Can you work these out from the drawing? Everything is in mm from the part's minimum corner. A direction names the side the tool comes from. Give positions to 0.01 mm unless a question says otherwise; leave off trailing zeros. Write each loop counter-clockwise with the first axis right and the second up, starting at its lowest first coordinate (ties: lowest second). Pieces come first, ordered by that corner, then holes. Notation, with made-up numbers: (71.5, -10) -> (99.5, -10) arc R26 ccw to (99.5, 21) -> close; hole circle Ø2 at (-14, 19.5). An arc over 180 degrees is marked (long way). Return JSON: item names as keys, results as strings.
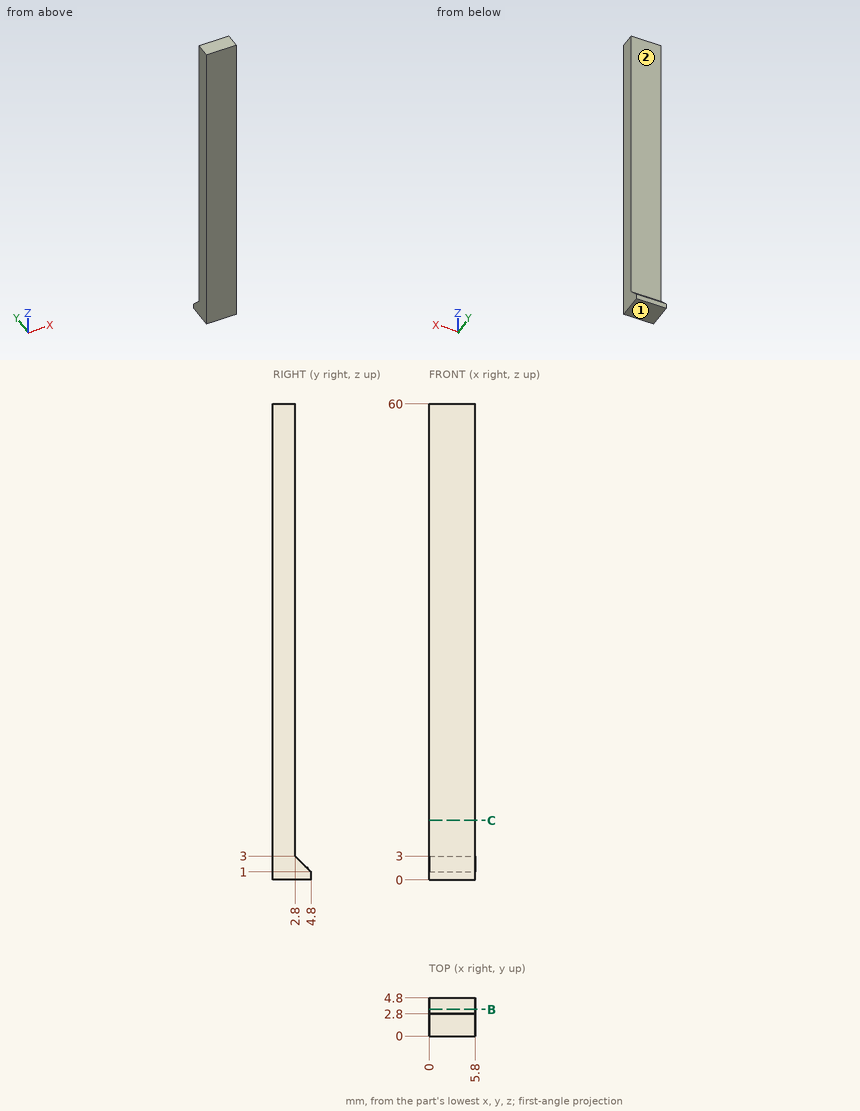
1. Suppose I cut it at B-B, the plane y = 3.35. List the corners of the cut face in (x, z) for me, and give its area (3 significant figures).
Taken from the geometry:
{"outline": "(0, 0) -> (5.8, 0) -> (5.8, 2.45) -> (0, 2.45) -> close", "area": "14.2 mm²"}
2. If I drill on line 1 (Y direction, x = 5.25, z = 41); line 2 (Z direction, x = 3.8, y = 4.65), over which ranges is the centre line in solid material (lowest first)? Write a range as [from, to].
Taken from the geometry:
{"line 1": "y = [0, 2.8]", "line 2": "z = [0, 1.15]"}
3. Suppose I cut it at C-C, the plane z = 7.5. List the corners of the cut face in (x, y) for me.
Taken from the geometry:
{"outline": "(0, 0) -> (5.8, 0) -> (5.8, 2.8) -> (0, 2.8) -> close"}
4. For pin 1 Ø3 at (x, z) = (5, 9.5) entering from +Y, with a flat end and sliding along its axis, tell me the tip position at first contact or that it passes through.
Taken from the geometry:
{"pin 1": "stops at y = 2.8"}
5. Which directions (+Z, -Z, +X, -X, +Y, -Y) give clear straight access to the entire face, cutting with the end or side of a thin tool? Please do the marked faces 1 and 2.
Taken from the geometry:
{"face 1": "-Z, +X, -X, +Y, -Y", "face 2": "+Z, +X, -X, +Y"}
